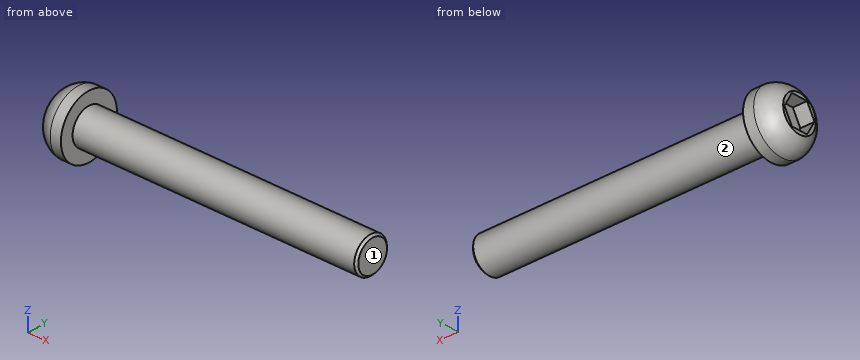
from build123d import *

# Parameters (mm, degrees)
CHAMFER1_SIZE      = 0.3
CUT_EXTRUDE1_DEPTH = 2


with BuildPart() as part:
    # Sketch1 → Revolve1 (revolve)
    with BuildSketch(Plane.XY):
        with BuildLine():
            Line((0, 0), (44, 0))
            Line((44, 0), (44, 2.5))
            Line((44, 2.5), (4, 2.5))
            Line((4, 2.5), (4, 4.3))
            Line((4, 4.3), (2.5, 4.3))
            ThreePointArc((2.5, 4.3), (1.027835828, 3.70856135), (0, 2.5))
            Line((0, 2.5), (0, 0))
        make_face()
    revolve(axis=Axis((0, 0, 0), (1, 0, 0)))

    # Chamfer1
    chamfer1_edges = [part.edges().sort_by_distance(p)[0] for p in [
        (44, -2.5, 0),
    ]]
    chamfer(chamfer1_edges, length=CHAMFER1_SIZE)

    # Sketch2 → Cut-Extrude1 (cut)
    with BuildSketch(Plane.ZY):
        Polygon((0, 2.309401077), (-2, 1.154700538), (-2, -1.154700538), (0, -2.309401077), (2, -1.154700538), (2, 1.154700538), align=None)
    extrude(amount=-CUT_EXTRUDE1_DEPTH, mode=Mode.SUBTRACT)


solid = part.part
The model under review builds one solid part; all positions refer to its coordinate system, in mm. Face numbers are marked on the shaded views. A direction names the side the tool comes from. Give positions to 0.01 mm unless a question says otherwise; leave off trailing zeros. Write each loop counter-clockwise with the first axis right and the second up, starting at its lowest first coordinate (ties: lowest second). Pieces come first, ordered by that corner, then holes.
1. Wall thickness on L1, parallel to X at y = -0.75, z = -0.25; L2, parallel to Z at x = 28.5, y = 1.5: over which ranges is each line inside the solid? List them lowest first.
2. Add section A-A, the plane x = 12. Write out the cut boundary in (y, z), plus the area to 3 significant figures.
3. Tool access review of the marked faces 1 and 2: name each direction out of +Z, -Z, +X, -X, +Y, -Y from which nothing blocks a thin tool from reaching the whole face with its end or side.
4. For P1, Ø1, axis at y = -3.5, z = -1.5, coming from the -X side; P2, Ø2, axis at y = 0.5, z = -0.5, coming from the -X side; P3, Ø0.6, axis at x = 1, y = -0.5, coming from the -Z side; P4, Ø5, axis at x = 5.5, y = -2, coming from the +Z side, all flat-tipped, find the tip position at first contact; note any pin that passes through.
Worked answers:
1. L1: x = 2 to 44
1. L2: z = -2 to 2
2. outline: circle Ø5 at (0, 0)
2. area: 19.6 mm2
3. face 1: +Z, -Z, +X, +Y, -Y
3. face 2: +X
4. P1: stops at x = 0.57
4. P2: stops at x = 2
4. P3: stops at z = -3.86
4. P4: stops at z = 4.3
